```python
from build123d import *

# Parameters (mm, degrees)
SZKIC1_R                    = 10
DODANIE_WYCI_GNI_CIE2_DEPTH = 750
SZKIC3_R                    = 8
WYTNIJ_WYCI_GNI_CIE1_DEPTH  = 751
SZKIC4_R                    = 3
WYTNIJ_WYCI_GNI_CIE2_DEPTH  = 11


with BuildPart() as part:
    # Szkic1 → Dodanie-wyciągnięcie2 (new body)
    with BuildSketch(Plane.XY):
        Circle(SZKIC1_R)
    extrude(amount=DODANIE_WYCI_GNI_CIE2_DEPTH)

    # Szkic3 → Wytnij-wyciągnięcie1 (cut, through all)
    with BuildSketch(Plane.XY.offset(750)):
        Circle(SZKIC3_R)
    extrude(amount=-WYTNIJ_WYCI_GNI_CIE1_DEPTH, mode=Mode.SUBTRACT)

    # Szkic4 → Wytnij-wyciągnięcie2 (cut, symmetric)
    with BuildSketch(Plane(origin=(0, 0, 0), x_dir=(1, 0, 0), z_dir=(0, 1, 0))):
        with Locations((0, -7.5)):
            Circle(SZKIC4_R)
    wytnij_wyci_gni_cie2 = extrude(amount=WYTNIJ_WYCI_GNI_CIE2_DEPTH, both=True, mode=Mode.SUBTRACT)

    # Mirror1: Wytnij-wyciągnięcie2 across plane
    add(wytnij_wyci_gni_cie2.mirror(Plane.XY.offset(375)), mode=Mode.SUBTRACT)


solid = part.part
```
For this review, take the finished solid that the model builds, in its own axes (mm). Coordinates: 2 decimals unless noted, no trailing zeros. Order: outer loops, then holes, each group sorted by start corner. A loop starts at its lowest first (then second) coordinate and runs counter-clockwise, first axis right, second up. Notation, with made-up numbers: (-35.75, 72.5) -> (4.25, 72.5) arc R30 ccw to (4.25, 101.5) -> close; hole circle Ø10 at (11, 11.25). An arc over 180 degrees is marked (long way). Use CSV: the item, a comma, the result in double quotes. Start each with the question number.
Item 1: We need section B-B, the plane z = 671. Give the boundary of the cut face in (x, y).
Item 2: We need section A-A, the plane y = 0. Give the boundary of the cut face in (x, z), then the cut area to 3 significant figures.
Item 3: Insertion check: pin 1 (6 mm diameter, centred on x = 5.5, y = -3, fed in from -Z); pin 2 (4 mm diameter, centred on y = 4, z = 640.5, fed in from +X); pin 3 (2 mm diameter, centred on x = 6, z = 254.5, fed in from +Y); pin 4 (2 mm diameter, centred on x = 6.5, z = 628, fed in from -Y). Each pin has a flat end and moves straight along its axis. Give the tip position at first contact, or say it passes through.
Item 4: Wall thickness on probe 1 along Z at (x, y) = (0, -8.2); probe 2 along Y at (x, z) = (0, 500.5); probe 3 along X at (y, z) = (1.5, 679.5): over which ranges is each line inside the solid? List them lowest first.
Item 5: Draft analysis for pull direction X (two halves, no side actions). For faces 1 (the face through (-2.17, -9.76, 369.75)), 2 (the face through (-1.73, -7.81, 380.25)), 3 (the face through (0, 8.2, 0)), state which applies: pulls with the +X half, pulls with the -X half, needs draft (parallel to the pull), parting line crosses it, or undercut.
Derived:
1,outline,"circle Ø20 at (0, 0); hole circle Ø16 at (0, 0)"
2,outline,"(-10, 0) -> (-8, 0) -> (-8, 750) -> (-10, 750) -> close; (8, 0) -> (10, 0) -> (10, 750) -> (8, 750) -> close"
2,area,"3,000 mm^2"
3,pin 1,"stops at z = 0"
3,pin 2,"stops at x = 9.8"
3,pin 3,"stops at y = 8.66"
3,pin 4,"stops at y = -8.35"
4,probe 1,"z = 0 to 4.5, 10.5 to 739.5, 745.5 to 750"
4,probe 2,"y = -10 to -8, 8 to 10"
4,probe 3,"x = -9.89 to -7.86, 7.86 to 9.89"
5,face 1,"parting line crosses it"
5,face 2,"undercut"
5,face 3,"needs draft"
